Autodesk Inventor part; units mm, degrees
ref_plane "YZ Plane" through (0, 0, 0) normal (1, 0, 0) x (0, 1, 0)
ref_plane "XZ Plane" through (0, 0, 0) normal (0, 1, 0) x (-1, 0, 0)
ref_plane "XY Plane" through (0, 0, 0) normal (0, 0, 1) x (1, 0, 0)
sketch "Sketch1" plane through (0, 0, 0) normal (0, 0, 1) x (1, 0, 0)
  line L0 (0, 0) -> (165.1, 0)
  line L1 (165.1, 0) -> (165.1, 50.8)
  line L2 (165.1, 50.8) -> (0, 50.8)
  line L3 (0, 50.8) -> (0, 0)
  dimension "d0" = 165.1
  dimension "d1" = 50.8
extrude "Extrusion1" add sketch "Sketch1" along normal blind 6.35
sketch "Sketch3" plane through (0, 0, 6.35) normal (0, 0, 1) x (1, 0, 0)
  line L0 (39.6875, 25.4) -> (125.4125, 25.4)
  line L1 (0, 0) -> (165.1, 0)
  line L2 (0, 50.8) -> (0, 0)
  line L3 (165.1, 50.8) -> (0, 50.8)
  line L4 (82.55, 50.8) -> (82.55, 0)
  line L5 (165.1, 0) -> (165.1, 50.8)
  dimension "d14" = 85.725
  dimension "d15" = 25.4
  dimension "d16" = 39.6875
  dimension "d33" = 165.1
  dimension "d34" = 39.6875
hole "Hole1" at (39.6875, 25.4, 6.35) at (125.4125, 25.4, 6.35) direction (0, 0, -1) diameter 4.1656 depth 6.35 tip angle 118 counterbore diameter 7.9502 counterbore depth 2.54
sketch "Sketch4" plane through (0, 0, 0) normal (0, 0, -1) x (-1, 0, 0)
  line L0 (-139.7, 12.7) -> (-25.4, 12.7) construction
  line L1 (-139.7, 9.525) -> (-25.4, 9.525)
  line L2 (-25.4, 15.875) -> (-139.7, 15.875)
  arc A0 (-139.7, 15.875) -> (-139.7, 9.525) centre (-139.7, 12.7) ccw
  arc A1 (-25.4, 9.525) -> (-25.4, 15.875) centre (-25.4, 12.7) ccw
  line L3 (0, 50.8) -> (0, 0)
  line L4 (-139.7, 38.1) -> (-25.4, 38.1) construction
  line L5 (-139.7, 34.925) -> (-25.4, 34.925)
  line L6 (-25.4, 41.275) -> (-139.7, 41.275)
  arc A2 (-139.7, 41.275) -> (-139.7, 34.925) centre (-139.7, 38.1) ccw
  arc A3 (-25.4, 34.925) -> (-25.4, 41.275) centre (-25.4, 38.1) ccw
  line L7 (-165.1, 50.8) -> (0, 50.8)
  point P0 (-82.55, 12.7)
  point P1 (-82.55, 38.1)
  dimension "d24" = 6.35
  dimension "d25" = 25.4
  dimension "d26" = 114.3
  dimension "d27" = 6.35
  dimension "d28" = 25.4
  dimension "d29" = 12.7
  dimension "d32" = 114.3
extrude "Extrusion3" cut sketch "Sketch4" against normal blind 6.35
sketch "Sketch5" plane through (0, 0, 0) normal (0, 0, -1) x (-1, 0, 0)
  circle A0 centre (-39.6875, 25.4) radius 2.0828
  circle A1 centre (-125.4125, 25.4) radius 2.0828
  point P0 (0, 0)
hole "Hole2" at (39.6875, 25.4, 0) at (125.4125, 25.4, 0) direction (0, 0, 1) diameter 9.525 depth 2.54
properties part number "ps bottom"
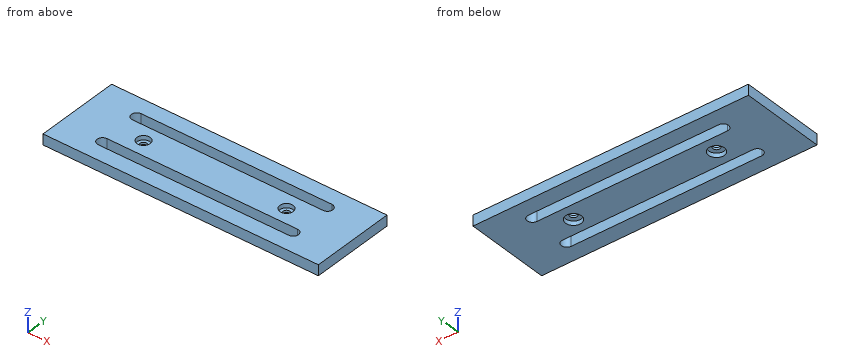
Input: part model. Units: mm. Frame: model coordinates. Coordinates: 2 decimals unless noted, no trailing zeros. Loops run counter-clockwise (first coordinate to the right, second up) from the corner with the lowest first, then second, coordinate; pieces in that order, holes last. Notation, with made-up numbers: (-13.5, 83) - (10.5, 83) arc R27 ccw to (10.5, 120) - close; hole circle Ø1 at (6.25, 71). An arc over 180 degrees is marked (long way). Answer in a Markdown table with one row per item.
(1) Cut plane B-B on x = 119. Output: boundary loops of the cut face in (y, z) (3 decimals), plus the area to 3 significant figures.
Model answer:
| item | result |
|---|---|
| outline | (0, 0) - (9.525, 0) - (9.525, 6.35) - (0, 6.35) - close; (15.875, 0) - (34.925, 0) - (34.925, 6.35) - (15.875, 6.35) - close; (41.275, 0) - (50.8, 0) - (50.8, 6.35) - (41.275, 6.35) - close |
| area | 242 mm² |
(2) Cut plane D-D on z = 5. Count the separate pieces of the cut face and the enclosed holes in it, plus the area to 3 significant figures.
Model answer:
| item | result |
|---|---|
| separate pieces | 1 |
| enclosed holes | 4 |
| area | 6,770 mm² |
(3) Material intervals for L1, parallel to Y at x = 30, z = 2 (3 decimals); L2, parallel to X at y = 25.4, z = 4.5; L3, parallel to X at y = 25.5, z = 1, sorted ascending. Write a range as from..to.
Model answer:
| item | result |
|---|---|
| L1 | y = 0..9.525, 15.875..34.925, 41.275..50.8 |
| L2 | x = 0..35.71, 43.66..121.44, 129.39..165.1 |
| L3 | x = 0..34.93, 44.45..120.65, 130.17..165.1 |
(4) Cut plane C-C on y = 25.4. Output: boundary loops of the cut face in (x, z) (3 decimals), plus the area to 3 significant figures.
Model answer:
| item | result |
|---|---|
| outline | (0, 0) - (34.925, 0) - (34.925, 2.54) - (37.605, 2.54) - (37.605, 3.81) - (35.712, 3.81) - (35.712, 6.35) - (0, 6.35) - close; (41.77, 2.54) - (44.45, 2.54) - (44.45, 0) - (120.65, 0) - (120.65, 2.54) - (123.33, 2.54) - (123.33, 3.81) - (121.437, 3.81) - (121.437, 6.35) - (43.663, 6.35) - (43.663, 3.81) - (41.77, 3.81) - close; (127.495, 2.54) - (130.175, 2.54) - (130.175, 0) - (165.1, 0) - (165.1, 6.35) - (129.388, 6.35) - (129.388, 3.81) - (127.495, 3.81) - close |
| area | 949 mm² |
(5) Pin query (flat end, axial travel): P1, Ø1, axis at x = 114, z = 5, coming from the -Y side; P2, Ø5.5, axis at x = 39.69, y = 25.4, coming from the +Z side; P3, Ø7, axis at x = 39.69, y = 25.4, coming from the -Z side; P4, Ø3.5, axis at x = 125.41, y = 25.4, coming from the +Z side. Return the tip coordinate at first contact, or that it passes through.
Model answer:
| item | result |
|---|---|
| P1 | stops at y = 0 |
| P2 | stops at z = 3.81 |
| P3 | stops at z = 2.54 |
| P4 | passes through |
(6) Cut plane A-A on y = 12.7. Output: boundary loops of the cut face in (x, z) (3 decimals), plus the area to 3 significant figures.
Model answer:
| item | result |
|---|---|
| outline | (0, 0) - (22.225, 0) - (22.225, 6.35) - (0, 6.35) - close; (142.875, 0) - (165.1, 0) - (165.1, 6.35) - (142.875, 6.35) - close |
| area | 282 mm² |
